Input: part model. Units: mm. Frame: model coordinates. A direction names the side the tool comes from. Coordinates: 2 decimals unless noted, no trailing zeros. Write each loop counter-clockwise with the first axis right and the second up, starting at its lowest first coordinate (ties: lowest second). Pieces come first, ordered by that corner, then holes. Notation, with made-up numbers: M 4.5,-14.75 L 22.5,-14.75 A26 cw 22.5,7.25 Z; hole C 62,-15 d7. An arc over 180 degrees is marked long. Use CSV: the item, a comma, the result in double quotes.
Solid Edge part; units mm, degrees
sketch "Sketch1" plane through (0, 0, 0) normal (0, 0, 1) x (1, 0, 0)
  circle A0 centre (0, 0) radius 4
  circle A1 centre (0, 0) radius 1.15
extrude "Protrusion1" add sketch "Sketch1" along normal blind 5.6
sketch "Sketch2" plane through (0, 0, 5.6) normal (0, 0, 1) x (1, 0, 0)
  circle A0 centre (0, 0) radius 2.275
extrude "ExtrudedCutout_1" cut sketch "Sketch2" against normal blind 2.75
sketch "Sketch3" plane through (0, 0, 0) normal (0, 0, -1) x (0, 1, 0)
  circle A0 centre (0, 0) radius 3.1
extrude "ExtrudedCutout_2" cut sketch "Sketch3" against normal blind 2
sketch "Sketch4" plane through (0, 0, 0) normal (0, 0, -1) x (-1, 0, 0)
  circle A0 centre (-10, 0) radius 0.8
  circle A1 centre (10, 0) radius 0.8
  circle A2 centre (12.5, 0) radius 0.8
  circle A3 centre (15, 0) radius 0.8
  circle A4 centre (-12.5, 0) radius 0.8
  circle A5 centre (-15, 0) radius 0.8
  line L0 (-15.1, 2.498) -> (-0.124, 3.0975)
  arc A6 (-0.124, 3.0975) -> (-0.124, -3.0975) centre (0, 0) ccw
  line L1 (-15.1, -2.498) -> (-0.124, -3.0975)
  arc A7 (-15.1, -2.498) -> (-15.1, 2.498) centre (-15, 0) cw
  line L2 (15.1, 2.498) -> (0.124, 3.0975)
  arc A8 (0.124, -3.0975) -> (0.124, 3.0975) centre (0, 0) ccw
  line L3 (15.1, -2.498) -> (0.124, -3.0975)
  arc A9 (15.1, -2.498) -> (15.1, 2.498) centre (15, 0) ccw
extrude "ExtrudedProtrusion_2" add sketch "Sketch4" against normal blind 2
1. Material intervals for line 1 (Y direction, x = -15, z = 1.3); line 2 (X direction, y = 0, z = 2.4); line 3 (Y direction, x = 0, z = 1), sorted ascending. Write a range as [from, to].
Resolved:
line 1,"y = [-2.5, -0.8], [0.8, 2.5]"
line 2,"x = [-4, -1.15], [1.15, 4]"
line 3,"y = [-4, -3.1], [3.1, 4]"
2. Section D-D (x = 7.5). Return loops of the section in (y, z).
Resolved:
outline,"M -2.8,0 L 2.8,0 L 2.8,2 L -2.8,2 Z"
3. Section B-B (x = -10). Return loops of the section in (y, z), then the cut area to 3 significant figures.
Resolved:
outline,"M -2.7,0 L -0.8,0 L -0.8,2 L -2.7,2 Z; M 0.8,0 L 2.7,0 L 2.7,2 L 0.8,2 Z"
area,"7.61 mm^2"
4. Mould query, pull axis X, two halves, no side actions, for faces 1 (the flat face through (-10, -1, 2)), 2 (the cylindrical face through (10.59, 0.54, 0.99)), 3 (the cylindrical face through (-17.5, -0.1, 1)). Classes: pulls with the +X half, pulls with the -X half, needs draft (parallel to the pull), parting line crosses it, or undercut.
Resolved:
face 1,"needs draft"
face 2,"undercut"
face 3,"pulls with the -X half"
5. Section C-C (y = 0). State how many separate pieces and enclosed holes the cut face has, then the cut area to 3 significant figures.
Resolved:
separate pieces,"8"
enclosed holes,"0"
area,"52.7 mm^2"
6. Section A-A (x = 0). Return loops of the section in (y, z) (3 decimals), then the cut area to 3 significant figures.
Resolved:
outline,"M -4,0 L -3.1,0 L -3.1,2 L -1.15,2 L -1.15,2.85 L -2.275,2.85 L -2.275,5.6 L -4,5.6 Z; M 1.15,2 L 3.1,2 L 3.1,0 L 4,0 L 4,5.6 L 2.275,5.6 L 2.275,2.85 L 1.15,2.85 Z"
area,"17.9 mm^2"
7. Access query for faces 4 (the flat face through (-1, 1, 2.85)), 5 (the cylindrical face through (-3.026, -0.672, 0.986)), 6 (the cylindrical face through (-0.91, 0.7, 2.42)). Directions: +Z, -Z, +X, -X, +Y, -Y. A direction counts if a zero-diameter tool reaches every point of the face in a straight line with its end or side. Return the directions, or none.
Resolved:
face 4,"+Z"
face 5,"-Z"
face 6,"+Z, -Z"
8. Contact query for flat-ended pins moving along their axis: pin 1 Ø2.5 at (x, y) = (15, 0) entering from +Z; pin 2 Ø1.5 at (x, z) = (-4, 1.5) entering from +Y; pin 3 Ø4 at (x, y) = (-12.5, 0) entering from -Z; pin 4 Ø2.5 at (x, y) = (0, 0) entering from +Z. Output: stop coordinate, or through.
Resolved:
pin 1,"stops at z = 2"
pin 2,"stops at y = 2.97"
pin 3,"stops at z = 0"
pin 4,"stops at z = 2.85"
